from build123d import *

# Parameters (mm, degrees)
SKETCH1_W            = 30.48
SKETCH1_H            = 31.75
BOSS_EXTRUDE1_DEPTH  = 3.556
BOSS_EXTRUDE2_DEPTH  = 12.7
SKETCH4_W            = 69.596
SKETCH4_H            = 73.406
BOSS_EXTRUDE3_DEPTH  = 3.556
BOSS_EXTRUDE5_DEPTH  = 12.7
MIRROR2_COPY_1_DEPTH = 12.7
MIRROR4_COPY_1_DEPTH = 12.7
FILLET5_R            = 1.778
SKETCH6_R            = 1.6
CUT_EXTRUDE1_DEPTH   = 80.692069935
BOSS_EXTRUDE7_REACH  = 82.336
SKETCH9_W            = 1.524
SKETCH9_H            = 35.306
SKETCH9_H_2          = 2.794
SKETCH9_W_2          = 34.036
SKETCH10_R           = 3.175
CUT_EXTRUDE2_DEPTH   = 2.54
BOSS_EXTRUDE8_DEPTH  = 5.08


with BuildPart() as part:
    # Sketch1 → Boss-Extrude1 (new body)
    with BuildSketch(Plane(origin=(0, 0, 0), x_dir=(1, 0, 0), z_dir=(0, 1, 0))):
        with Locations((15.24, 15.875)):
            Rectangle(SKETCH1_W, SKETCH1_H)
    extrude(amount=BOSS_EXTRUDE1_DEPTH)

    # Sketch2 → Boss-Extrude2 (add)
    with BuildSketch(Plane(origin=(0, 3.556, 0), x_dir=(1, 0, 0), z_dir=(0, 1, 0))):
        with BuildLine():
            Line((25.4, 6.35), (5.08, 6.35))
            ThreePointArc((5.08, 6.35), (15.24, 1.27), (25.4, 6.35))
        make_face()
        with BuildLine():
            ThreePointArc((25.4, 25.4), (15.24, 30.48), (5.08, 25.4))
            Line((5.08, 25.4), (25.4, 25.4))
        make_face()
    boss_extrude2 = extrude(amount=BOSS_EXTRUDE2_DEPTH)

    # Sketch4 → Boss-Extrude3 (add)
    with BuildSketch(Plane(origin=(0, 3.556, 0), x_dir=(1, 0, 0), z_dir=(0, 1, 0))):
        with Locations((33.02, -3.175)):
            Rectangle(SKETCH4_W, SKETCH4_H)
    extrude(amount=-BOSS_EXTRUDE3_DEPTH)

    # Sketch8 → Boss-Extrude5 (add)
    with BuildSketch(Plane(origin=(0, 3.556, 0), x_dir=(1, 0, 0), z_dir=(0, 1, 0))):
        Polygon((-1.778, 33.528), (-1.778, 27.178), (-1.778, 4.572), (-1.778, -1.778), (32.258, -1.778), (32.258, 33.528), align=None)
        Polygon((0, 27.178), (0, 31.75), (30.48, 31.75), (30.48, 0), (0, 0), (0, 4.572), align=None, mode=Mode.SUBTRACT)
    boss_extrude5 = extrude(amount=BOSS_EXTRUDE5_DEPTH)

    # Mirror1: Boss-Extrude5 across plane
    add(boss_extrude5.mirror(Plane(origin=(0, 0, 3.175), x_dir=(1, 0, 0), z_dir=(0, 0, -1))))

    # Mirror2: Boss-Extrude5 across plane
    add(boss_extrude5.mirror(Plane(origin=(33.02, 0, 0), x_dir=(0, 0, 1), z_dir=(1, 0, 0))))

    # Mirror2 copy 1 sketch → Mirror2 copy 1 (add)
    with BuildSketch(Plane(origin=(66.04, 3.556, 6.35), x_dir=(-1, 0, 0), z_dir=(0, 1, 0))):
        Polygon((-1.778, 33.528), (-1.778, 27.178), (-1.778, 4.572), (-1.778, -1.778), (32.258, -1.778), (32.258, 33.528), align=None)
        Polygon((0, 27.178), (0, 31.75), (30.48, 31.75), (30.48, 0), (0, 0), (0, 4.572), align=None, mode=Mode.SUBTRACT)
    extrude(amount=MIRROR2_COPY_1_DEPTH)

    # Mirror3: Boss-Extrude2 across plane
    add(boss_extrude2.mirror(Plane(origin=(0, 0, 3.175), x_dir=(1, 0, 0), z_dir=(0, 0, -1))))

    # Mirror4: Boss-Extrude2 across plane
    add(boss_extrude2.mirror(Plane(origin=(33.02, 0, 0), x_dir=(0, 0, 1), z_dir=(1, 0, 0))))

    # Mirror4 copy 1 sketch → Mirror4 copy 1 (add)
    with BuildSketch(Plane(origin=(66.04, 3.556, 6.35), x_dir=(-1, 0, 0), z_dir=(0, 1, 0))):
        with BuildLine():
            Line((25.4, 6.35), (5.08, 6.35))
            ThreePointArc((5.08, 6.35), (15.24, 1.27), (25.4, 6.35))
        make_face()
        with BuildLine():
            ThreePointArc((25.4, 25.4), (15.24, 30.48), (5.08, 25.4))
            Line((5.08, 25.4), (25.4, 25.4))
        make_face()
    extrude(amount=MIRROR4_COPY_1_DEPTH)

    # Fillet5
    fillet5_edges = [part.edges().sort_by_distance(p)[0] for p in [
        (15.24, 16.256, -1.27),
        (15.24, 16.256, 7.62),
        (15.24, 16.256, 36.83),
        (50.8, 16.256, 7.62),
        (50.8, 16.256, 36.83),
        (50.8, 16.256, -1.27),
        (50.8, 16.256, -30.48),
        (15.24, 16.256, -30.48),
    ]]
    fillet(fillet5_edges, radius=FILLET5_R)

    # Sketch6 → Cut-Extrude1 (cut, through all)
    with BuildSketch(Plane(origin=(0, 3.556, 0), x_dir=(1, 0, 0), z_dir=(0, 1, 0))):
        with Locations(Location((61.5442, 17.402175, 0), (0, 0, 270))):
            Circle(SKETCH6_R)
        with Locations(Location((4.4958, 17.402175, 0), (0, 0, 270))):
            Circle(SKETCH6_R)
        with Locations(Location((4.4958, -23.753445, 0), (0, 0, 270))):
            Circle(SKETCH6_R)
        with Locations(Location((61.5442, -23.753445, 0), (0, 0, 270))):
            Circle(SKETCH6_R)
    extrude(amount=-CUT_EXTRUDE1_DEPTH, mode=Mode.SUBTRACT)

    # Sketch9 → Boss-Extrude7 (add, up to next)
    with BuildSketch(Plane(origin=(0, 16.256, 0), x_dir=(1, 0, 0), z_dir=(0, 1, 0)), mode=Mode.PRIVATE) as boss_extrude7_sk1:
        with Locations((33.02, 15.875)):
            Rectangle(SKETCH9_W, SKETCH9_H)
    boss_extrude7_tool1 = extrude(boss_extrude7_sk1.sketch, amount=-BOSS_EXTRUDE7_REACH, mode=Mode.PRIVATE) - part.part
    # Sketch9 → Boss-Extrude7 (add, up to next)
    with BuildSketch(Plane(origin=(0, 16.256, 0), x_dir=(1, 0, 0), z_dir=(0, 1, 0)), mode=Mode.PRIVATE) as boss_extrude7_sk2:
        with Locations((33.02, -22.225)):
            Rectangle(SKETCH9_W, SKETCH9_H)
    boss_extrude7_tool2 = extrude(boss_extrude7_sk2.sketch, amount=-BOSS_EXTRUDE7_REACH, mode=Mode.PRIVATE) - part.part
    # Sketch9 → Boss-Extrude7 (add, up to next)
    with BuildSketch(Plane(origin=(0, 16.256, 0), x_dir=(1, 0, 0), z_dir=(0, 1, 0)), mode=Mode.PRIVATE) as boss_extrude7_sk3:
        with Locations((33.02, -3.175)):
            Rectangle(SKETCH9_W, SKETCH9_H_2)
    boss_extrude7_tool3 = extrude(boss_extrude7_sk3.sketch, amount=-BOSS_EXTRUDE7_REACH, mode=Mode.PRIVATE) - part.part
    # Sketch9 → Boss-Extrude7 (add, up to next)
    with BuildSketch(Plane(origin=(0, 16.256, 0), x_dir=(1, 0, 0), z_dir=(0, 1, 0)), mode=Mode.PRIVATE) as boss_extrude7_sk4:
        with Locations((50.8, -3.175)):
            Rectangle(SKETCH9_W_2, SKETCH9_H_2)
    boss_extrude7_tool4 = extrude(boss_extrude7_sk4.sketch, amount=-BOSS_EXTRUDE7_REACH, mode=Mode.PRIVATE) - part.part
    # Sketch9 → Boss-Extrude7 (add, up to next)
    with BuildSketch(Plane(origin=(0, 16.256, 0), x_dir=(1, 0, 0), z_dir=(0, 1, 0)), mode=Mode.PRIVATE) as boss_extrude7_sk5:
        with Locations((15.24, -3.175)):
            Rectangle(SKETCH9_W_2, SKETCH9_H_2)
    boss_extrude7_tool5 = extrude(boss_extrude7_sk5.sketch, amount=-BOSS_EXTRUDE7_REACH, mode=Mode.PRIVATE) - part.part
    add(boss_extrude7_tool1.solids().sort_by_distance((33.02, 16.256, -15.875))[0])
    add(boss_extrude7_tool2.solids().sort_by_distance((33.02, 16.256, 22.225))[0])
    add(boss_extrude7_tool3.solids().sort_by_distance((33.02, 16.256, 3.175))[0])
    add(boss_extrude7_tool4.solids().sort_by_distance((50.8, 16.256, 3.175))[0])
    add(boss_extrude7_tool5.solids().sort_by_distance((15.24, 16.256, 3.175))[0])

    # Sketch10 → Cut-Extrude2 (cut)
    with BuildSketch(Plane(origin=(0, 3.556, 0), x_dir=(1, 0, 0), z_dir=(0, 1, 0))):
        with Locations(Location((61.5442, 17.402175, 0), (0, 0, 270))):
            Circle(SKETCH10_R)
        with Locations(Location((4.4958, 17.402175, 0), (0, 0, 270))):
            Circle(SKETCH10_R)
        with Locations(Location((4.4958, -23.753445, 0), (0, 0, 270))):
            Circle(SKETCH10_R)
        with Locations(Location((61.5442, -23.753445, 0), (0, 0, 270))):
            Circle(SKETCH10_R)
    extrude(amount=-CUT_EXTRUDE2_DEPTH, mode=Mode.SUBTRACT)

    # Sketch12 → Boss-Extrude8 (add)
    with BuildSketch(Plane(origin=(0, 16.256, 0), x_dir=(1, 0, 0), z_dir=(0, 1, 0))):
        Polygon((-1.778, 25.4), (0, 25.4), (0, 31.75), (30.48, 31.75), (30.48, 0), (0, 0), (0, 6.35), (-1.778, 6.35), (-1.778, -12.7), (0, -12.7), (0, -6.35), (30.48, -6.35), (30.48, -38.1), (0, -38.1), (0, -31.75), (-1.778, -31.75), (-1.778, -39.878), (67.818, -39.878), (67.818, -31.75), (66.04, -31.75), (66.04, -38.1), (35.56, -38.1), (35.56, -6.35), (66.04, -6.35), (66.04, -12.7), (67.818, -12.7), (67.818, 6.35), (66.04, 6.35), (66.04, 0), (35.56, 0), (35.56, 31.75), (66.04, 31.75), (66.04, 25.4), (67.818, 25.4), (67.818, 33.528), (-1.778, 33.528), align=None)
    extrude(amount=BOSS_EXTRUDE8_DEPTH)


solid = part.part
Design review of the part built by this model. Coordinates are the model's own, in mm. A direction names the side the tool comes from. Give positions to 0.01 mm unless a question says otherwise; leave off trailing zeros. Order: outer loops, then holes, each group sorted by start corner. A loop starts at its lowest first (then second) coordinate and runs counter-clockwise, first axis right, second up.
1. Add section A-A, the plane x = 38. State the section outline as (y, z) points, then the cut area to 3 significant figures.
Solution:
outline: (0, -33.53) - (21.34, -33.53) - (21.34, -31.75) - (3.56, -31.75) - (3.56, 0) - (21.34, 0) - (21.34, 6.35) - (3.56, 6.35) - (3.56, 38.1) - (21.34, 38.1) - (21.34, 39.88) - (0, 39.88) - close
area: 437 mm2
2. Add section D-D, the plane z = 24.5. State the section outline as (x, y) points.
Solution:
outline: (-1.78, 0) - (3.08, 0) - (3.08, 1.02) - (1.41, 1.02) - (1.41, 3.56) - (0, 3.56) - (0, 16.26) - (-1.78, 16.26) - close; (5.91, 0) - (60.13, 0) - (60.13, 1.02) - (58.46, 1.02) - (58.46, 3.56) - (35.56, 3.56) - (35.56, 21.34) - (30.48, 21.34) - (30.48, 3.56) - (7.58, 3.56) - (7.58, 1.02) - (5.91, 1.02) - close; (62.96, 0) - (67.82, 0) - (67.82, 16.26) - (66.04, 16.26) - (66.04, 3.56) - (64.63, 3.56) - (64.63, 1.02) - (62.96, 1.02) - close
3. To check wall thickness, follow L1, parallel to Z at x = 18.5, y = 17; L2, parallel to X at y = 10, z = -8.5; L3, parallel to X at y = 12, z = -29. State the ranges of each line that lie inside material, in increasing order.
Solution:
L1: z = -33.53 to -31.75, 0 to 6.35, 38.1 to 39.88
L2: x = -1.78 to 0, 30.48 to 35.56, 66.04 to 67.82
L3: x = -1.78 to 0, 9.29 to 21.19, 30.48 to 35.56, 44.85 to 56.75, 66.04 to 67.82
4. Mouldability with a two-part tool opening along X and no side actions: class faces 1 (the flat face through (33, 11, 39.878)), 2 (the cylindrical face through (3.28, 2.3, -14.47)) as +X half, -X half, draft (parallel to the pull), parting line (faces both ways), or undercut.
Solution:
face 1: draft
face 2: undercut
5. Tool access review of faces 3 (the flat face through (-1, 19, -25.4)), 4 (the flat face through (60, 1.016, -16)): name each direction out of +Z, -Z, +X, -X, +Y, -Y from which nothing blocks a thin tool from reaching the whole face with its end or side.
Solution:
face 3: -X, +Y
face 4: +Y
6. Add section C-C, the plane y = 12.75. State how many separate pieces and enclosed holes the cut face has, then the cut area to 3 significant figures.
Solution:
separate pieces: 9
enclosed holes: 4
area: 1,810 mm2
7. Add section B-B, the plane z = 14. State the section outline as (x, y) points, then the cut area to 3 significant figures.
Solution:
outline: (-1.78, 0) - (67.82, 0) - (67.82, 16.26) - (66.04, 16.26) - (66.04, 3.56) - (35.56, 3.56) - (35.56, 21.34) - (30.48, 21.34) - (30.48, 3.56) - (0, 3.56) - (0, 16.26) - (-1.78, 16.26) - close
area: 383 mm2
8. For pin 1 Ø4 at (x, z) = (61.54, 23.75) entering from +Y; pin 2 Ø15 at (x, z) = (56, -10) entering from +Y; pin 3 Ø6 at (x, z) = (25, 10) entering from +Y, all flat-tipped, find the tip position at first contact; note any pin that passes through.
Solution:
pin 1: stops at y = 1.02
pin 2: stops at y = 16.26
pin 3: stops at y = 16.23
